Geometry check sheet. Reference: the model listing, model coordinates, mm. Face numbers are marked on the shaded views. A direction names the side the tool comes from. Coordinates: 2 decimals unless noted, no trailing zeros. Write each loop counter-clockwise with the first axis right and the second up, starting at its lowest first coordinate (ties: lowest second). Pieces come first, ordered by that corner, then holes. Notation, with made-up numbers: (22, -32.5) -> (57, -32.5) arc R24 ccw to (57, -17.5) -> close; hole circle Ø10 at (61.5, 74). An arc over 180 degrees is marked (long way). Answer as CSV lines item,"result".
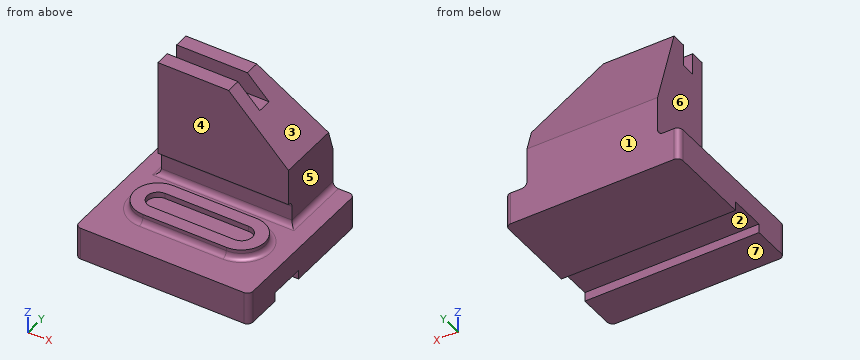
```python
from build123d import *

# Parameters (mm, degrees)
F0_W      = 96
F0_H      = 90
F1_DEPTH  = 18
F2_W      = 72
F2_H      = 38
F4_DEPTH  = 67
F6_DEPTH  = 38
F7_W      = 8
F7_H      = 12
F8_DEPTH  = 51.001
F10_DEPTH = 72.001
F11_W     = 20
F11_H     = 5
F12_DEPTH = 96
F14_W     = 46
F14_H     = 26
F15_DEPTH = 5
F17_DEPTH = 3
F18_W     = 3
F18_H     = 14
F19_DEPTH = 72
F20_R     = 2.99999


# Not quite as in the source:
# - a fillet or chamfer is up to 0.001 mm smaller than in the source, because OpenCascade refuses the exact size


with BuildPart() as f1:
    # F0 (on Top) → F1 (new body)
    with BuildSketch(Plane.XY):
        with Locations((48, 45)):
            Rectangle(F0_W, F0_H)
    extrude(amount=F1_DEPTH)

    # F2 (on face) → F4 (join, through all)
    with BuildSketch(Plane.XY.offset(18)):
        with Locations((48, 71)):
            Rectangle(F2_W, F2_H)
    extrude(amount=F4_DEPTH)

    # F5 (on face) → F6 (cut)
    with BuildSketch(Plane.XZ.offset(-52)):
        Polygon((84, 52), (84, 85), (51, 85), align=None)
    extrude(amount=-F6_DEPTH, mode=Mode.SUBTRACT)

    # F7 (on face) → F8 (cut, through all)
    with BuildSketch(Plane(origin=(12, 0, 0), x_dir=(0, -1, 0), z_dir=(-1, 0, 0))):
        with Locations((-64, 79)):
            Rectangle(F7_W, F7_H)
    extrude(amount=-F8_DEPTH, mode=Mode.SUBTRACT)

    # F9 (on face) → F10 (cut, through all)
    with BuildSketch(Plane(origin=(12, 0, 0), x_dir=(0, -1, 0), z_dir=(-1, 0, 0))):
        Polygon((-76, 85), (-90, 85), (-90, 40), align=None)
    extrude(amount=-F10_DEPTH, mode=Mode.SUBTRACT)

    # F11 (on face) → F12 (cut, through all)
    with BuildSketch(Plane.YZ.offset(96)):
        with Locations((32, 2.5)):
            Rectangle(F11_W, F11_H)
    extrude(amount=-F12_DEPTH, mode=Mode.SUBTRACT)

    # F14 (on face) → F15 (join)
    with BuildSketch(Plane.XY.offset(18)):
        with Locations((48, 32)):
            Rectangle(F14_W, F14_H)
        with BuildLine():
            Line((25, 19), (25, 45))
            ThreePointArc((25, 45), (12, 32), (25, 19))
        make_face()
        with BuildLine():
            ThreePointArc((71, 19), (84, 32), (71, 45))
            Line((71, 45), (71, 19))
        make_face()
    extrude(amount=F15_DEPTH)

    # F16 (on face) → F17 (cut)
    with BuildSketch(Plane.XY.offset(23)):
        with BuildLine():
            ThreePointArc((25, 38), (19, 32), (25, 26))
            Line((25, 26), (71, 26))
            ThreePointArc((71, 26), (77, 32), (71, 38))
            Line((71, 38), (25, 38))
        make_face()
    extrude(amount=-F17_DEPTH, mode=Mode.SUBTRACT)

    # F18 (on face) → F19 (cut, through all)
    with BuildSketch(Plane.YZ.offset(84)):
        with Locations((53.5, 25)):
            Rectangle(F18_W, F18_H)
    extrude(amount=-F19_DEPTH, mode=Mode.SUBTRACT)

    # F20 (radius 3 in the source; OpenCascade refuses exactly that, so slightly less here)
    f20_edges = [f1.edges().sort_by_distance(p)[0] for p in [
        (48, 19, 18),
        (48, 55, 18),
        (48, 55, 32),
        (0, 0, 9),
        (96, 0, 9),
        (96, 90, 9),
        (0, 90, 9),
        (84, 72.5, 18),
        (12, 72.5, 18),
    ]]
    fillet(f20_edges, radius=F20_R)


solid = f1.part
```
Item 1: Depth check by flat-ended pin: pin 1 Ø25 at (y, z) = (75.5, 33.5) entering from +X; pin 2 Ø2 at (x, y) = (76.5, 60.5) entering from +Z; pin 3 Ø5 at (x, z) = (45, 67) entering from -Y. Enter the tip coordinate at first touch or a pass-through.
Responses:
pin 1,"stops at x = 84"
pin 2,"stops at z = 60.5"
pin 3,"stops at y = 52"
Item 2: Thickness scan on probe 1 along Z at (x, y) = (69, 51.5); probe 2 along Z at (x, y) = (28, 54); probe 3 along Z at (x, y) = (33, 30.5). Record the ranges inside material, lowest first.
Responses:
probe 1,"z = 0 to 18"
probe 2,"z = 0 to 18.76, 31.24 to 85"
probe 3,"z = 5 to 20"
Item 3: Cross-section at D-D, the plane y = 6. Record the cut outline in (x, z), plus the area to 3 significant figures.
Responses:
outline,"(0, 0) -> (96, 0) -> (96, 18) -> (0, 18) -> close"
area,"1,730 mm2"
Item 4: Release check for a two-part mould opening along Y. For the marked faces 1, 2, 3 and 4 record: +Y half, -Y half, draft (parallel to the pull), parting line (faces both ways), or undercut.
Responses:
face 1,"+Y half"
face 2,"undercut"
face 3,"draft"
face 4,"-Y half"
Item 5: Set-up check for the marked faces 5, 6 and 7: record each of +Z, -Z, +X, -X, +Y, -Y from which the full face is reachable in a straight line by a thin tool's end or side.
Responses:
face 5,"+Z, +X, +Y, -Y"
face 6,"+Z, -X, +Y, -Y"
face 7,"-Z, +X, -X, +Y, -Y"
Item 6: Cross-section at C-C, the plane z = 36.5. Record the cut outline in (x, y).
Responses:
outline,"(12, 52) -> (84, 52) -> (84, 90) -> (12, 90) -> close"
Item 7: Cross-section at A-A, the plane y = 32. Record the cut outline in (x, z).
Responses:
outline,"(0, 5) -> (96, 5) -> (96, 18) -> (87, 18) arc R3 cw to (84, 21) -> (84, 23) -> (77, 23) -> (77, 20) -> (19, 20) -> (19, 23) -> (12, 23) -> (12, 21) arc R3 cw to (9, 18) -> (0, 18) -> close"
